from build123d import *

# Parameters (mm, degrees)
F0_W     = 146.05
F0_H     = 76.2
F1_DEPTH = 12.954
F2_W     = 39.624
F2_H     = 3.302
F3_DEPTH = 76.201
F4_W     = 66.802
F4_H     = 3.302
F5_DEPTH = 76.201
F6_R     = 12.7
F7_R     = 6.35
F9_DEPTH = 9.653


with BuildPart() as f1:
    # F0 (on Top) → F1 (new body)
    with BuildSketch(Plane.XY):
        with Locations((73.025, 38.1)):
            Rectangle(F0_W, F0_H)
    extrude(amount=F1_DEPTH)

    # F2 (on face) → F3 (cut, through all)
    with BuildSketch(Plane.XZ):
        with Locations((126.238, 11.303)):
            Rectangle(F2_W, F2_H)
        with Locations((19.812, 11.303)):
            Rectangle(F2_W, F2_H)
    extrude(amount=-F3_DEPTH, mode=Mode.SUBTRACT)

    # F4 (on face) → F5 (cut, through all)
    with BuildSketch(Plane.XZ):
        with Locations((73.025, 1.651)):
            Rectangle(F4_W, F4_H)
    extrude(amount=-F5_DEPTH, mode=Mode.SUBTRACT)

    # F6
    f6_edges = [f1.edges().sort_by_distance(p)[0] for p in [
        (0, 0, 4.826),
        (0, 76.2, 4.826),
        (146.05, 76.2, 4.826),
        (146.05, 0, 4.826),
    ]]
    fillet(f6_edges, radius=F6_R)

    # F8 (on face) + F7 (on face) → F9 (cut, through all)
    with BuildSketch(Plane.XY.offset(9.652)):
        with BuildLine():
            Line((133.35, 63.5), (139.7, 63.5))
            ThreePointArc((139.7, 63.5), (128.859872, 67.990128), (133.35, 57.15))
            Line((133.35, 57.15), (133.35, 63.5))
        make_face()
        with BuildLine():
            ThreePointArc((133.35, 57.15), (137.840128, 59.009872), (139.7, 63.5))
            Line((139.7, 63.5), (133.35, 63.5))
            Line((133.35, 63.5), (133.35, 57.15))
        make_face()
        with BuildLine():
            ThreePointArc((139.7, 12.7), (137.840128, 17.190128), (133.35, 19.05))
            ThreePointArc((133.35, 19.05), (128.859872, 8.209872), (139.7, 12.7))
        make_face()
    with BuildSketch(Plane.XY.offset(9.652)):
        with Locations((12.7, 63.5)):
            Circle(F7_R)
        with BuildLine():
            Line((12.7, 12.7), (12.7, 6.35))
            ThreePointArc((12.7, 6.35), (17.190128, 8.209872), (19.05, 12.7))
            ThreePointArc((19.05, 12.7), (12.7, 19.05), (6.35, 12.7))
            Line((6.35, 12.7), (12.7, 12.7))
        make_face()
        with BuildLine():
            ThreePointArc((6.35, 12.7), (8.209872, 8.209872), (12.7, 6.35))
            Line((12.7, 6.35), (12.7, 12.7))
            Line((12.7, 12.7), (6.35, 12.7))
        make_face()
    extrude(amount=-F9_DEPTH, mode=Mode.SUBTRACT)


solid = f1.part
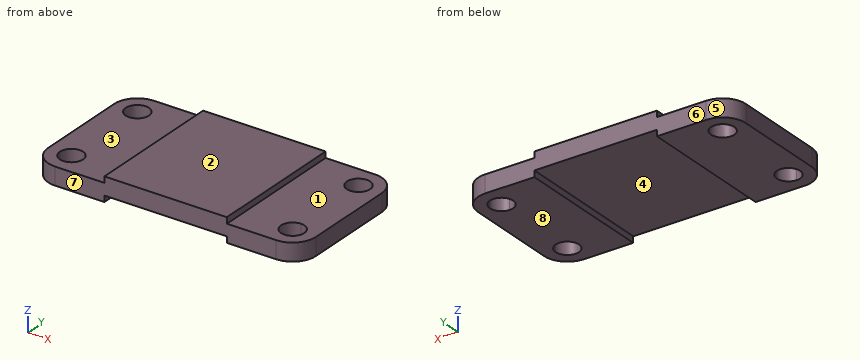
Work out the finished part from the listing and answer in its coordinate system (mm). Face numbers are marked on the shaded views. A direction names the side the tool comes from. Round coordinates to 2 decimals unless told otherwise and drop trailing zeros. Order: outer loops, then holes, each group sorted by start corner. A loop starts at its lowest first (then second) coordinate and runs counter-clockwise, first axis right, second up. Notation, with made-up numbers: M 4.5,-32.5 L 10.5,-32.5 A17 cw 10.5,-7.5 Z; hole C -28,17 d10. An arc over 180 degrees is marked long. Put each result on its own line as item: value. Start each with the question number.
Q1. Section A-A, the plane y = 45 is taken. Write down the section's boundary in (x, z).
Q2. Flat-ended cylindrical pins translate along their axes: pin 1 (3.5 mm diameter, centred on y = 28, z = 12, fed in from +X); pin 2 (2 mm diameter, centred on x = 117.5, y = 28.5, fed in from +Z); pin 3 (8 mm diameter, centred on x = 65.5, y = 24, fed in from -Z). Find the tip coordinate at first contact, or state that the pin passes through.
Q3. Section B-B, the plane y = 15 is taken. Write down the section's boundary in (x, z), and give its area (3 significant figures).
Q4. Section D-D, the plane x = 80 is taken. Write down the section's boundary in (y, z).
Q5. Section C-C, the plane x = 17 is taken. Write down the section's boundary in (y, z), and give its area (3 significant figures).
Q6. Straight lines are drawn through the part: L1, parallel to X at y = 12.7, z = 2.5; L2, parallel to X at y = 12.7, z = 6.5; L3, parallel to Y at x = 12.7, z = 3.5. For each, find the intervals that lie inside material, in ascending order. Write a range as [from, to].
Q7. A tool of negligible diameter and unlimited length cuts with its end or side. For the marked faces 1, 2, 3, 4 and 5, from which of +Z, -Z, +X, -X, +Y, -Y can it reach the whole face along a straight path? Write none if from no direction.
Q8. For a pull along Y with two mould halves and no side action, classify the marked faces 6, 7 and 8 as pulls with the +Y half, pulls with the -Y half, needs draft (parallel to the pull), parting line crosses it, or undercut.
Findings below:
1. outline: M 0,0 L 39.62,0 L 39.62,3.3 L 106.43,3.3 L 106.43,0 L 146.05,0 L 146.05,9.65 L 106.43,9.65 L 106.43,12.95 L 39.62,12.95 L 39.62,9.65 L 0,9.65 Z
2. pin 1: stops at x = 106.43
2. pin 2: stops at z = 9.65
2. pin 3: stops at z = 3.3
3. outline: M 0,0 L 6.78,0 L 6.78,9.65 L 0,9.65 Z; M 18.62,0 L 39.62,0 L 39.62,3.3 L 106.43,3.3 L 106.43,0 L 127.43,0 L 127.43,9.65 L 106.43,9.65 L 106.43,12.95 L 39.62,12.95 L 39.62,9.65 L 18.62,9.65 Z; M 139.27,0 L 146.05,0 L 146.05,9.65 L 139.27,9.65 Z
3. area: 1,180 mm^2
4. outline: M 0,3.3 L 76.2,3.3 L 76.2,12.95 L 0,12.95 Z
5. outline: M 0,0 L 8.03,0 L 8.03,9.65 L 0,9.65 Z; M 17.37,0 L 58.83,0 L 58.83,9.65 L 17.37,9.65 Z; M 68.17,0 L 76.2,0 L 76.2,9.65 L 68.17,9.65 Z
5. area: 555 mm^2
6. L1: x = [0, 6.35], [19.05, 39.62], [106.43, 127], [139.7, 146.05]
6. L2: x = [0, 6.35], [19.05, 127], [139.7, 146.05]
6. L3: y = [0, 6.35], [19.05, 57.15], [69.85, 76.2]
7. face 1: +Z, +X, +Y, -Y
7. face 2: +Z, +X, -X, +Y, -Y
7. face 3: +Z, -X, +Y, -Y
7. face 4: -Z, +Y, -Y
7. face 5: +Z, -Z, -X, +Y
8. face 6: pulls with the +Y half
8. face 7: pulls with the -Y half
8. face 8: needs draft
